```python
from build123d import *

# Parameters (mm, degrees)
SKETCH1_R           = 2.25
BOSS_EXTRUDE1_DEPTH = 6.2
SKETCH2_OUTSIDE_W   = 8.276
SKETCH2_OUTSIDE_H   = 8.276
SKETCH2_OUTSIDE_R   = 1.65
CUT_EXTRUDE1_DEPTH  = 1.3
SKETCH3_R           = 1.25
CUT_EXTRUDE2_DEPTH  = 7.2
CHAMFER1_SIZE       = 0.2


with BuildPart() as part:
    # Sketch1 → Boss-Extrude1 (new body)
    with BuildSketch(Plane.XY):
        Circle(SKETCH1_R)
    extrude(amount=-BOSS_EXTRUDE1_DEPTH)

    # Sketch2 outside → Cut-Extrude1 (cut)
    with BuildSketch(Plane(origin=(0, 0, -6.2), x_dir=(-1, 0, 0), z_dir=(0, 0, -1))):
        Rectangle(SKETCH2_OUTSIDE_W, SKETCH2_OUTSIDE_H)
        Circle(SKETCH2_OUTSIDE_R, mode=Mode.SUBTRACT)
    extrude(amount=-CUT_EXTRUDE1_DEPTH, mode=Mode.SUBTRACT)

    # Sketch3 → Cut-Extrude2 (cut, through all)
    with BuildSketch(Plane.XY):
        Circle(SKETCH3_R)
    extrude(amount=-CUT_EXTRUDE2_DEPTH, mode=Mode.SUBTRACT)

    # Chamfer1
    chamfer1_edges = [part.edges().sort_by_distance(p)[0] for p in [
        (1.65, 0, -6.2),
    ]]
    chamfer(chamfer1_edges, length=CHAMFER1_SIZE)


solid = part.part
```
The model under review builds one solid part; all positions refer to its coordinate system, in mm. A direction names the side the tool comes from. Coordinates: 2 decimals unless noted, no trailing zeros. Order: outer loops, then holes, each group sorted by start corner. A loop starts at its lowest first (then second) coordinate and runs counter-clockwise, first axis right, second up. Notation, with made-up numbers: (30, -26.75) -> (82, -26.75) arc R18 cw to (82, -13.75) -> close; hole circle Ø3 at (13.25, 9). An arc over 180 degrees is marked (long way). Answer in a Markdown table with one row per item. Add a question column.
Item 1: Clearance check with flat-ended pins moving along their axes: pin 1 (1.3 mm diameter, centred on x = 1, y = 0.5, fed in from -Z); pin 2 (1.5 mm diameter, centred on x = 0, y = 0, fed in from +Z). State where each tip first meets the part, or that it passes through.
Item 2: We need section A-A on x = 0. Write out the cut boundary in (y, z).
Item 3: Machinability: for faces 4 (the flat face through (0, 2, -4.9)), 5 (the cylindrical face through (-0.29, 2.23, -2.42)), which of the approach directions +Z, -Z, +X, -X, +Y, -Y give a long, thin tool a straight path to every point of the face, cutting with its end or side? Answer none if there is none.
Item 4: To check wall thickness, follow probe 1 along Y at (x, z) = (0, -2.75); probe 2 along Z at (x, y) = (-2, 0.4); probe 3 along Y at (x, z) = (1.1, -0.75). State the ranges of each line that lie inside material, in increasing order.
Item 5: We need section C-C on z = -4.75. Write out the cut boundary in (x, y), plus the area to 3 significant figures.
Item 6: We need section D-D on y = -1.8. Write out the cut boundary in (x, z).
Item 7: Mouldability with a two-part tool opening along Y and no side actions: class faces 1 (the flat face through (1, -1, 0)), 2 (the cylindrical face through (-0.27, -1.22, -3.06)), 3 (the cylindrical face through (1.216, 1.115, -5.458)) as +Y half, -Y half, draft (parallel to the pull), parting line (faces both ways), or undercut.
Final values:
| question | item | result |
|---|---|---|
| 1 | pin 1 | stops at z = -6.2 |
| 1 | pin 2 | passes through |
| 2 | outline | (-2.25, -4.9) -> (-1.65, -4.9) -> (-1.65, -6) -> (-1.45, -6.2) -> (-1.25, -6.2) -> (-1.25, 0) -> (-2.25, 0) -> close; (1.25, -6.2) -> (1.45, -6.2) -> (1.65, -6) -> (1.65, -4.9) -> (2.25, -4.9) -> (2.25, 0) -> (1.25, 0) -> close |
| 3 | face 4 | -Z |
| 3 | face 5 | +Z, -Z |
| 4 | probe 1 | y = -2.25 to -1.25, 1.25 to 2.25 |
| 4 | probe 2 | z = -4.9 to 0 |
| 4 | probe 3 | y = -1.96 to -0.59, 0.59 to 1.96 |
| 5 | outline | circle Ø4.5 at (0, 0); hole circle Ø2.5 at (0, 0) |
| 5 | area | 11.0 mm2 |
| 6 | outline | (-1.35, -4.9) -> (1.35, -4.9) -> (1.35, 0) -> (-1.35, 0) -> close |
| 7 | face 1 | draft |
| 7 | face 2 | undercut |
| 7 | face 3 | parting line |
